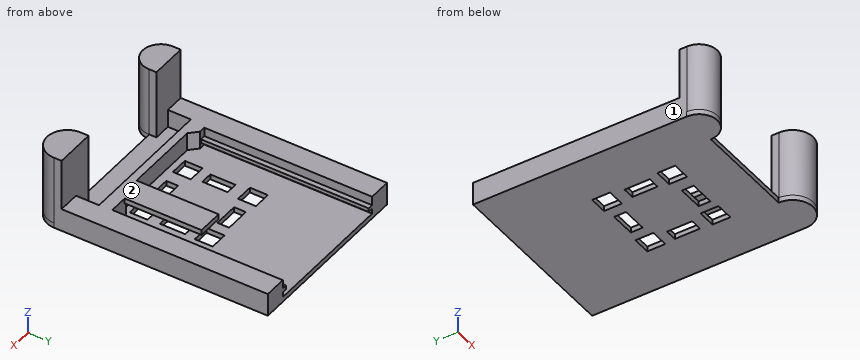
from build123d import *

# Parameters (mm, degrees)
BOSS_EXTRUDE1_DEPTH = 7
SKETCH3_W           = 1.5
SKETCH3_H           = 65.5
BOSS_EXTRUDE2_DEPTH = 2
SKETCH4_W           = 1.5
SKETCH4_H           = 66.5
BOSS_EXTRUDE3_DEPTH = 2
SKETCH7_W           = 10
SKETCH7_H           = 33.446163333
BOSS_EXTRUDE6_DEPTH = 2
BOSS_EXTRUDE7_DEPTH = 2
BOSS_EXTRUDE8_DEPTH = 20
SKETCH15_W          = 7
SKETCH15_H          = 7
CUT_EXTRUDE4_DEPTH  = 2
SKETCH16_W          = 4.633871769
SKETCH16_H          = 9.84697751
SKETCH16_W_2        = 9.84697751
SKETCH16_H_2        = 4.63387177
SKETCH16_H_3        = 9.846977511
CUT_EXTRUDE5_DEPTH  = 2


with BuildPart() as part:
    # Sketch2 → Boss-Extrude1 (new body)
    with BuildSketch(Plane.XY):
        with BuildLine():
            Line((70, 0), (70, 71.493036289))
            Line((70, 71.493036289), (61.25, 71.493036289))
            Line((61.25, 71.493036289), (61.25, 4.993036289))
            Line((61.25, 4.993036289), (53.25, 4.993036289))
            Line((53.25, 4.993036289), (51.365136631, 2.993036289))
            Line((51.365136631, 2.993036289), (14.25, 2.993036289))
            Line((14.25, 2.993036289), (11.25, 5.993036289))
            Line((11.25, 5.993036289), (8.75, 5.993036289))
            Line((8.75, 5.993036289), (8.75, 71.493036289))
            Line((8.75, 71.493036289), (0, 71.493036289))
            Line((0, 71.493036289), (0, 0))
            Line((0, 0), (0, -12))
            ThreePointArc((0, -12), (7.120138309, -19.120138309), (14.240276619, -12))
            Line((14.240276619, -12), (14.240276619, -9))
            Line((14.240276619, -9), (7.551059866, -9))
            Line((7.551059866, -9), (7.551059866, 0))
            Line((7.551059866, 0), (61.551059866, 0))
            Line((61.551059866, 0), (61.551059866, -9))
            Line((61.551059866, -9), (54.143055629, -9))
            Line((54.143055629, -9), (54.143055629, -12))
            ThreePointArc((54.143055629, -12), (62.071527814, -19.928472186), (70, -12))
            Line((70, -12), (70, 0))
        make_face()
    extrude(amount=BOSS_EXTRUDE1_DEPTH)

    # Sketch3 → Boss-Extrude2 (add)
    with BuildSketch(Plane(origin=(8.75, 0, 0), x_dir=(0, 0, -1), z_dir=(1, 0, 0))):
        with Locations((-2.75, 38.743036289)):
            Rectangle(SKETCH3_W, SKETCH3_H)
    extrude(amount=BOSS_EXTRUDE2_DEPTH)

    # Sketch4 → Boss-Extrude3 (add)
    with BuildSketch(Plane.ZY.offset(-61.25)):
        with Locations((2.75, 38.243036289)):
            Rectangle(SKETCH4_W, SKETCH4_H)
    extrude(amount=BOSS_EXTRUDE3_DEPTH)

    # Sketch7 → Boss-Extrude6 (add)
    with BuildSketch(Plane.XY.offset(7)):
        with Locations((49.00753408, 18.276918333)):
            Rectangle(SKETCH7_W, SKETCH7_H)
    extrude(amount=-BOSS_EXTRUDE6_DEPTH)

    # Sketch8 → Boss-Extrude7 (add)
    with BuildSketch(Plane(origin=(0, 0, 0), x_dir=(-1, 0, 0), z_dir=(0, 0, -1))):
        with BuildLine():
            Line((-70, 71.493036289), (0, 71.493036289))
            Line((0, 71.493036289), (0, -11.821263414))
            ThreePointArc((0, -11.821263414), (-7.120138309, -19.120135173), (-14.240276619, -11.821263414))
            Line((-14.240276619, -11.821263414), (-54.143055629, -11.821263414))
            ThreePointArc((-54.143055629, -11.821263414), (-61.981146501, -19.928975841), (-70, -12))
            Line((-70, -12), (-70, 71.493036289))
        make_face()
    extrude(amount=BOSS_EXTRUDE7_DEPTH)

    # Sketch14 → Boss-Extrude8 (add)
    with BuildSketch(Plane.XY.offset(7)):
        with BuildLine():
            Line((14.240276619, -12), (14.240276619, -9))
            Line((14.240276619, -9), (0, -9))
            Line((0, -9), (0, -12))
            ThreePointArc((0, -12), (7.120138309, -19.120138309), (14.240276619, -12))
        make_face()
        with BuildLine():
            Line((54.143055629, -12), (54.143055629, -9))
            Line((54.143055629, -9), (70, -9))
            Line((70, -9), (70, -12))
            ThreePointArc((70, -12), (62.071527814, -19.928472186), (54.143055629, -12))
        make_face()
    extrude(amount=BOSS_EXTRUDE8_DEPTH)

    # Sketch15 → Cut-Extrude4 (cut)
    with BuildSketch(Plane(origin=(0, 0, -2), x_dir=(-1, 0, 0), z_dir=(0, 0, -1))):
        with Locations((-48.294388032, 8.963448797)):
            Rectangle(SKETCH15_W, SKETCH15_H)
        with Locations((-48.294388032, 34.373848797)):
            Rectangle(SKETCH15_W, SKETCH15_H)
        with Locations((-22.874388032, 8.963448797)):
            Rectangle(SKETCH15_W, SKETCH15_H)
        with Locations((-22.874388032, 34.373848797)):
            Rectangle(SKETCH15_W, SKETCH15_H)
    extrude(amount=-CUT_EXTRUDE4_DEPTH, mode=Mode.SUBTRACT)

    # Sketch16 → Cut-Extrude5 (cut)
    with BuildSketch(Plane(origin=(0, 0, -2), x_dir=(-1, 0, 0), z_dir=(0, 0, -1))):
        with Locations((-49.007648907, 21.901962869)):
            Rectangle(SKETCH16_W, SKETCH16_H)
        with Locations((-35.672375834, 34.542330615)):
            Rectangle(SKETCH16_W_2, SKETCH16_H_2)
        with Locations((-36.367281161, 8.566689797)):
            Rectangle(SKETCH16_W_2, SKETCH16_H_2)
        with Locations((-23.032008088, 21.207057543)):
            Rectangle(SKETCH16_W, SKETCH16_H_3)
    extrude(amount=-CUT_EXTRUDE5_DEPTH, mode=Mode.SUBTRACT)


solid = part.part
Read the model definition and answer for the solid it produces. Units are mm, in the model's axes. Face numbers are marked on the shaded views. A direction names the side the tool comes from. Give positions to 0.01 mm unless a question says otherwise; leave off trailing zeros. Write each loop counter-clockwise with the first axis right and the second up, starting at its lowest first coordinate (ties: lowest second). Pieces come first, ordered by that corner, then holes. Notation, with made-up numbers: (70, 61.5) - (112, 61.5) arc R20 ccw to (112, 81.5) - close; hole circle Ø1 at (79.25, -23). An arc over 180 degrees is marked (long way). Return JSON: item names as keys, results as strings.
Q1. For the marked faces 1 and 2, determine the directions among +Z, -Z, +X, -X, +Y, -Y from which every point of the face is accessible in a straight line to the end or side of a thin tool.
Reply:
{"face 1": "+Z, -Z, -X, +Y, -Y", "face 2": "+Z, +X, -X, +Y"}
Q2. A cutting plane is placed at B-B, the plane z = 10.5. Determine the outline of the cut face in (x, y), and give its area (3 significant figures).
Reply:
{"outline": "(0, -12) arc R7.12 ccw to (14.24, -12) - (14.24, -9) - (0, -9) - close; (54.14, -12) arc R7.93 ccw to (70, -12) - (70, -9) - (54.14, -9) - close", "area": "269 mm²"}
Q3. A cutting plane is placed at D-D, the plane y = 42.5. Determine the outline of the cut face in (x, z), and give its area (4 significant figures).
Reply:
{"outline": "(0, -2) - (70, -2) - (70, 7) - (61.25, 7) - (61.25, 3.5) - (59.25, 3.5) - (59.25, 2) - (61.25, 2) - (61.25, 0) - (8.75, 0) - (8.75, 2) - (10.75, 2) - (10.75, 3.5) - (8.75, 3.5) - (8.75, 7) - (0, 7) - close", "area": "268.5 mm²"}
Q4. A cutting plane is placed at A-A, the plane x = 35.5. Determine the outline of the cut face in (y, z), and give its area (3 significant figures).
Reply:
{"outline": "(-11.82, -2) - (6.25, -2) - (6.25, 0) - (2.99, 0) - (2.99, 7) - (0, 7) - (0, 0) - (-11.82, 0) - close; (10.88, -2) - (32.23, -2) - (32.23, 0) - (10.88, 0) - close; (36.86, -2) - (71.49, -2) - (71.49, 0) - (36.86, 0) - close", "area": "169 mm²"}
Q5. A cutting plane is placed at C-C, the plane y = 29. Determine the outline of the cut face in (x, z), and give its area (4 significant figures).
Reply:
{"outline": "(0, -2) - (70, -2) - (70, 7) - (61.25, 7) - (61.25, 3.5) - (59.25, 3.5) - (59.25, 2) - (61.25, 2) - (61.25, 0) - (8.75, 0) - (8.75, 2) - (10.75, 2) - (10.75, 3.5) - (8.75, 3.5) - (8.75, 7) - (0, 7) - close; (44.01, 5) - (54.01, 5) - (54.01, 7) - (44.01, 7) - close", "area": "288.5 mm²"}
Q6. Given P1, Ø10, axis at x = 56.5, z = 20, coming from the -Y side; P2, Ø1, axis at x = 60.5, y = 28.5, coming from the +Z side; P3, Ø1, axis at y = 23, z = -1, coming from the -X side, each flat-ended and moving along its own axis, determine where each tip first touches the part or whether it passes through.
Reply:
{"P1": "y = -19.91", "P2": "z = 3.5", "P3": "x = 0"}
Q7. Consider line 1 along Z through (x, y) = (59.5, 32); line 2 along X through (y, z) = (36.5, 0.5); line 3 along Y through (x, z) = (22.5, 1). Determine where each line is inside the solid, lowest interval first. Write a range as [from, to].
Reply:
{"line 1": "[-2, 0], [2, 3.5]", "line 2": "[0, 8.75], [61.25, 70]", "line 3": "[0, 2.99]"}
